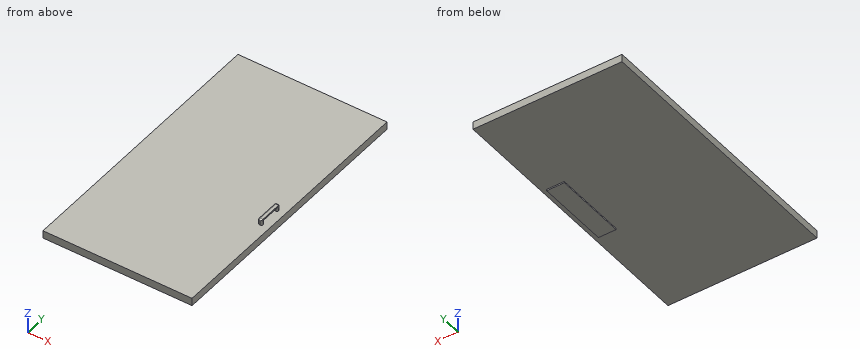
from build123d import *

# Parameters (mm, degrees)
BOSS_EXTRUDE2_DEPTH = 57.15
BOSS_EXTRUDE3_DEPTH = 44
CUT_EXTRUDE1_DEPTH  = 44
FILLET1_R           = 10
BOSS_EXTRUDE4_DEPTH = 10


with BuildPart() as part:
    # Sketch1 → Boss-Extrude2 (new body)
    with BuildSketch(Plane.XY):
        Polygon((0, 0), (0, 446.2018372120283), (-1100, 446.2018372120282), (-1100, -1585.7981627879717), (0, -1585.7981627879717), align=None)
    extrude(amount=BOSS_EXTRUDE2_DEPTH)

    # Sketch4 → Boss-Extrude3 (add)
    with BuildSketch(Plane.XY.offset(57.15)):
        Polygon((-79.99999999999993, -603.7981627879718), (-49.999999999999936, -603.7981627879718), (-49.999999999999915, -785.7981627879718), (-79.9999999999999, -785.7981627879718), align=None)
    extrude(amount=BOSS_EXTRUDE3_DEPTH)

    # Sketch5 → Cut-Extrude1 (cut)
    with BuildSketch(Plane.ZY.offset(80.00000000000003)):
        Polygon((83.14999999999999, -624.7981627879717), (57.150000000000006, -624.7981627879717), (57.15, -764.7981627879717), (83.15, -764.7981627879717), align=None)
    extrude(amount=-CUT_EXTRUDE1_DEPTH, mode=Mode.SUBTRACT)

    # Fillet1
    # the kernel refuses this fillet: 10 mm, written as the material it takes off along each edge
    with BuildSketch(Plane(origin=(-69.99999999999993, -613.7981627879718, 91.15), x_dir=(-1, -1.6e-16, 0), z_dir=(0, 1, 0))) as fillet1_piece_1_section:
        Polygon((0, 0), (FILLET1_R, 0), (FILLET1_R, FILLET1_R), (0, FILLET1_R), align=None)
    fillet1_piece_1 = extrude(amount=FILLET1_R, mode=Mode.PRIVATE)
    fillet1_piece_1 = fillet1_piece_1 - Plane(origin=(-69.99999999999993, -613.7981627879718, 91.15), x_dir=(0.7071067811865475, 0, -0.7071067811865475), z_dir=(0, 1, 0)) * Sphere(FILLET1_R, mode=Mode.PRIVATE)
    add(fillet1_piece_1, mode=Mode.SUBTRACT)
    with BuildSketch(Plane(origin=(-69.9999999999999, -775.7981627879718, 91.15), x_dir=(0, 0, 1), z_dir=(-1, -1.6e-16, 0))) as fillet1_piece_2_section:
        Polygon((0, 0), (FILLET1_R, 0), (FILLET1_R, -FILLET1_R), (0, -FILLET1_R), align=None)
    fillet1_piece_2 = extrude(amount=FILLET1_R, mode=Mode.PRIVATE)
    fillet1_piece_2 = fillet1_piece_2 - Plane(origin=(-69.9999999999999, -775.7981627879718, 91.15), x_dir=(0, 0.7071067811865475, -0.7071067811865475), z_dir=(-1, -1.6e-16, 0)) * Sphere(FILLET1_R, mode=Mode.PRIVATE)
    add(fillet1_piece_2, mode=Mode.SUBTRACT)
    with BuildSketch(Plane(origin=(-49.999999999999915, -785.7981627879718, 57.15), x_dir=(-1, 0, 0), z_dir=(0, 0, 1))) as fillet1_piece_3:
        with BuildLine():
            CenterArc((FILLET1_R, -FILLET1_R), FILLET1_R, 90, 90)
            Line((0, -FILLET1_R), (0, 0))
            Line((0, 0), (FILLET1_R, 0))
        make_face()
    extrude(amount=69, mode=Mode.SUBTRACT)
    with BuildSketch(Plane(origin=(-49.999999999999936, -603.7981627879718, 57.15), x_dir=(0, -1, 0), z_dir=(0, 0, 1))) as fillet1_piece_4:
        with BuildLine():
            CenterArc((FILLET1_R, -FILLET1_R), FILLET1_R, 90, 90)
            Line((0, -FILLET1_R), (0, 0))
            Line((0, 0), (FILLET1_R, 0))
        make_face()
    extrude(amount=69, mode=Mode.SUBTRACT)
    with BuildSketch(Plane(origin=(-79.99999999999993, -603.7981627879718, 57.15), x_dir=(1, 0, 0), z_dir=(0, 0, 1))) as fillet1_piece_5:
        with BuildLine():
            CenterArc((FILLET1_R, -FILLET1_R), FILLET1_R, 90, 90)
            Line((0, -FILLET1_R), (0, 0))
            Line((0, 0), (FILLET1_R, 0))
        make_face()
    extrude(amount=34.00000000000001, mode=Mode.SUBTRACT)
    with BuildSketch(Plane(origin=(-79.9999999999999, -785.7981627879718, 57.15), x_dir=(1, 0, 0), z_dir=(0, 0, 1))) as fillet1_piece_6:
        with BuildLine():
            CenterArc((FILLET1_R, FILLET1_R), FILLET1_R, 180, 90)
            Line((0, FILLET1_R), (0, 0))
            Line((0, 0), (FILLET1_R, 0))
        make_face()
    extrude(amount=34.00000000000001, mode=Mode.SUBTRACT)
    with BuildSketch(Plane(origin=(-69.99999999999993, -603.7981627879718, 101.15), x_dir=(0, 0, -1), z_dir=(1, 0, 0))) as fillet1_piece_7:
        with BuildLine():
            CenterArc((FILLET1_R, -FILLET1_R), FILLET1_R, 90, 90)
            Line((0, -FILLET1_R), (0, 0))
            Line((0, 0), (FILLET1_R, 0))
        make_face()
    extrude(amount=44.99999999999999, mode=Mode.SUBTRACT)
    with BuildSketch(Plane(origin=(-79.9999999999999, -775.7981627879718, 101.15), x_dir=(0, 0, -1), z_dir=(-1.6e-16, 1, 0))) as fillet1_piece_8:
        with BuildLine():
            CenterArc((FILLET1_R, -FILLET1_R), FILLET1_R, 90, 90)
            Line((0, -FILLET1_R), (0, 0))
            Line((0, 0), (FILLET1_R, 0))
        make_face()
    extrude(amount=162, mode=Mode.SUBTRACT)
    with BuildSketch(Plane(origin=(-24.999999999999915, -785.7981627879718, 101.15), x_dir=(0, 0, -1), z_dir=(-1, 0, 0))) as fillet1_piece_9:
        with BuildLine():
            CenterArc((FILLET1_R, -FILLET1_R), FILLET1_R, 90, 90)
            Line((0, -FILLET1_R), (0, 0))
            Line((0, 0), (FILLET1_R, 0))
        make_face()
    extrude(amount=44.999999999999986, mode=Mode.SUBTRACT)
    with BuildSketch(Plane(origin=(-79.99999999999991, -764.7981627879717, 57.15000000000002), x_dir=(1.42e-15, -1, 0), z_dir=(0, 0, 1))) as fillet1_piece_10:
        with BuildLine():
            CenterArc((FILLET1_R, FILLET1_R), FILLET1_R, 180, 89.99999999999989)
            Line((1.421e-14, FILLET1_R), (0, 0))
            Line((0, 0), (FILLET1_R, 0))
        make_face()
    extrude(amount=25.999999999999986, mode=Mode.SUBTRACT)
    with BuildSketch(Plane(origin=(-79.99999999999993, -624.7981627879717, 83.14999999999999), x_dir=(0, 1, 0), z_dir=(0, 0, -1))) as fillet1_piece_11:
        with BuildLine():
            CenterArc((FILLET1_R, FILLET1_R), FILLET1_R, 180, 90)
            Line((0, FILLET1_R), (0, 0))
            Line((0, 0), (FILLET1_R, 0))
        make_face()
    extrude(amount=25.999999999999986, mode=Mode.SUBTRACT)
    with BuildSketch(Plane(origin=(-79.99999999999991, -764.7981627879717, 83.15), x_dir=(1.42e-15, 1e-16, 1), z_dir=(-1.5e-16, 1, -1e-16))) as fillet1_piece_12:
        with BuildLine():
            CenterArc((FILLET1_R, FILLET1_R), FILLET1_R, 180, 89.99999999999989)
            Line((1.421e-14, FILLET1_R), (0, 0))
            Line((0, 0), (FILLET1_R, 0))
        make_face()
    extrude(amount=140, mode=Mode.SUBTRACT)
    with BuildSketch(Plane(origin=(-49.999999999999915, -764.7981627879717, 83.15), x_dir=(0, -1, 0), z_dir=(0, 0, -1))) as fillet1_piece_13:
        with BuildLine():
            CenterArc((FILLET1_R, FILLET1_R), FILLET1_R, 180, 90)
            Line((0, FILLET1_R), (0, 0))
            Line((0, 0), (FILLET1_R, 0))
        make_face()
    extrude(amount=26, mode=Mode.SUBTRACT)
    with BuildSketch(Plane(origin=(-49.999999999999936, -624.7981627879717, 57.150000000000006), x_dir=(0, 1, 0), z_dir=(0, 0, 1))) as fillet1_piece_14:
        with BuildLine():
            CenterArc((FILLET1_R, FILLET1_R), FILLET1_R, 180.00000000000003, 90)
            Line((0, FILLET1_R), (0, 0))
            Line((0, 0), (FILLET1_R, 0))
        make_face()
    extrude(amount=25.999999999999986, mode=Mode.SUBTRACT)
    with BuildSketch(Plane(origin=(-49.999999999999936, -624.7981627879717, 83.15), x_dir=(0, 1e-16, 1), z_dir=(1.2e-16, -1, 1e-16))) as fillet1_piece_15:
        with BuildLine():
            CenterArc((FILLET1_R, FILLET1_R), FILLET1_R, 180, 90)
            Line((0, FILLET1_R), (0, 0))
            Line((0, 0), (FILLET1_R, 0))
        make_face()
    extrude(amount=140, mode=Mode.SUBTRACT)
    with BuildSketch(Plane(origin=(-79.99999999999991, -764.7981627879717, 57.15000000000002), x_dir=(1.42e-15, -1, 0), z_dir=(0, 0, 1))) as fillet1_piece_16a_section:
        with BuildLine():
            CenterArc((FILLET1_R, FILLET1_R), FILLET1_R, 180, 89.99999999999989)
            Line((1.421e-14, FILLET1_R), (0, 0))
            Line((0, 0), (FILLET1_R, 0))
        make_face()
    fillet1_piece_16a = extrude(amount=50.999999999999986, mode=Mode.PRIVATE)
    fillet1_piece_16a = split(fillet1_piece_16a, bisect_by=Plane(origin=(-77.7360488573316, -767.0621139306398, 83.15), z_dir=(0, 1e-16, 1)), keep=Keep.TOP, mode=Mode.PRIVATE)
    with BuildSketch(Plane(origin=(-79.9999999999999, -789.7981627879717, 83.15), x_dir=(0, 1e-16, 1), z_dir=(-1.5e-16, 1, -1e-16))) as fillet1_piece_16b_section:
        with BuildLine():
            CenterArc((FILLET1_R, FILLET1_R), FILLET1_R, 180, 90)
            Line((0, FILLET1_R), (0, 0))
            Line((0, 0), (FILLET1_R, 0))
        make_face()
    fillet1_piece_16b = extrude(amount=165, mode=Mode.PRIVATE)
    fillet1_piece_16b = split(fillet1_piece_16b, bisect_by=Plane(origin=(-77.73604885733165, -764.7981627879717, 85.41395114266827), z_dir=(1.5e-16, -1, 0)), keep=Keep.TOP, mode=Mode.PRIVATE)
    fillet1_piece_16 = fillet1_piece_16a & fillet1_piece_16b
    add(fillet1_piece_16, mode=Mode.SUBTRACT)
    with BuildSketch(Plane(origin=(-79.99999999999991, -764.7981627879717, 83.15), x_dir=(1.42e-15, 1e-16, 1), z_dir=(-1.5e-16, 1, -1e-16))) as fillet1_piece_17a_section:
        with BuildLine():
            CenterArc((FILLET1_R, FILLET1_R), FILLET1_R, 180, 89.99999999999989)
            Line((1.421e-14, FILLET1_R), (0, 0))
            Line((0, 0), (FILLET1_R, 0))
        make_face()
    fillet1_piece_17a = extrude(amount=165, mode=Mode.PRIVATE)
    fillet1_piece_17a = split(fillet1_piece_17a, bisect_by=Plane(origin=(-77.73604885733167, -624.7981627879717, 85.41395114266825), z_dir=(-1.5e-16, 1, 0)), keep=Keep.TOP, mode=Mode.PRIVATE)
    with BuildSketch(Plane(origin=(-79.99999999999993, -624.7981627879717, 108.14999999999998), x_dir=(0, 1, 0), z_dir=(0, 0, -1))) as fillet1_piece_17b_section:
        with BuildLine():
            CenterArc((FILLET1_R, FILLET1_R), FILLET1_R, 180, 90)
            Line((0, FILLET1_R), (0, 0))
            Line((0, 0), (FILLET1_R, 0))
        make_face()
    fillet1_piece_17b = extrude(amount=50.999999999999986, mode=Mode.PRIVATE)
    fillet1_piece_17b = split(fillet1_piece_17b, bisect_by=Plane(origin=(-77.73604885733164, -622.5342116453035, 83.14999999999999), z_dir=(0, 1e-16, 1)), keep=Keep.TOP, mode=Mode.PRIVATE)
    fillet1_piece_17 = fillet1_piece_17a & fillet1_piece_17b
    add(fillet1_piece_17, mode=Mode.SUBTRACT)
    with BuildSketch(Plane(origin=(-49.999999999999936, -624.7981627879717, 83.15), x_dir=(0, 1e-16, 1), z_dir=(1.2e-16, -1, 1e-16))) as fillet1_piece_18a_section:
        with BuildLine():
            CenterArc((FILLET1_R, FILLET1_R), FILLET1_R, 180, 90)
            Line((0, FILLET1_R), (0, 0))
            Line((0, 0), (FILLET1_R, 0))
        make_face()
    fillet1_piece_18a = extrude(amount=165, mode=Mode.PRIVATE)
    fillet1_piece_18a = split(fillet1_piece_18a, bisect_by=Plane(origin=(-52.26395114266817, -764.7981627879717, 85.41395114266827), z_dir=(1.5e-16, -1, 0)), keep=Keep.TOP, mode=Mode.PRIVATE)
    with BuildSketch(Plane(origin=(-49.999999999999915, -764.7981627879717, 108.15), x_dir=(0, -1, 0), z_dir=(0, 0, -1))) as fillet1_piece_18b_section:
        with BuildLine():
            CenterArc((FILLET1_R, FILLET1_R), FILLET1_R, 180, 90)
            Line((0, FILLET1_R), (0, 0))
            Line((0, 0), (FILLET1_R, 0))
        make_face()
    fillet1_piece_18b = extrude(amount=51, mode=Mode.PRIVATE)
    fillet1_piece_18b = split(fillet1_piece_18b, bisect_by=Plane(origin=(-52.2639511426682, -767.0621139306397, 83.15), z_dir=(0, 1e-16, 1)), keep=Keep.TOP, mode=Mode.PRIVATE)
    fillet1_piece_18 = fillet1_piece_18a & fillet1_piece_18b
    add(fillet1_piece_18, mode=Mode.SUBTRACT)
    with BuildSketch(Plane(origin=(-49.999999999999936, -624.7981627879717, 57.150000000000006), x_dir=(0, 1, 0), z_dir=(0, 0, 1))) as fillet1_piece_19a_section:
        with BuildLine():
            CenterArc((FILLET1_R, FILLET1_R), FILLET1_R, 180.00000000000003, 90)
            Line((0, FILLET1_R), (0, 0))
            Line((0, 0), (FILLET1_R, 0))
        make_face()
    fillet1_piece_19a = extrude(amount=50.999999999999986, mode=Mode.PRIVATE)
    fillet1_piece_19a = split(fillet1_piece_19a, bisect_by=Plane(origin=(-52.26395114266823, -622.5342116453035, 83.14999999999999), z_dir=(0, 1e-16, 1)), keep=Keep.TOP, mode=Mode.PRIVATE)
    with BuildSketch(Plane(origin=(-49.999999999999936, -599.7981627879717, 83.14999999999999), x_dir=(0, 1e-16, 1), z_dir=(1.2e-16, -1, 1e-16))) as fillet1_piece_19b_section:
        with BuildLine():
            CenterArc((FILLET1_R, FILLET1_R), FILLET1_R, 179.99999999999997, 90)
            Line((0, FILLET1_R), (0, 0))
            Line((0, 0), (FILLET1_R, 0))
        make_face()
    fillet1_piece_19b = extrude(amount=165, mode=Mode.PRIVATE)
    fillet1_piece_19b = split(fillet1_piece_19b, bisect_by=Plane(origin=(-52.26395114266818, -624.7981627879717, 85.41395114266824), z_dir=(-1.5e-16, 1, 0)), keep=Keep.TOP, mode=Mode.PRIVATE)
    fillet1_piece_19 = fillet1_piece_19a & fillet1_piece_19b
    add(fillet1_piece_19, mode=Mode.SUBTRACT)

    # Sketch6 → Boss-Extrude4 (add)
    with BuildSketch(Plane(origin=(0, 0, 0), x_dir=(-1, 0, 0), z_dir=(0, 0, -1))):
        Polygon((34.99999999999994, -272.04870051020725), (164.99999999999986, -272.04870051020725), (165, -812.0487005102073), (35, -812.0487005102073), align=None)
    extrude(amount=BOSS_EXTRUDE4_DEPTH)


solid = part.part
CAD build for the part. Positions are in the model's coordinates, mm. Coordinates: 2 decimals unless noted, no trailing zeros. Write each loop counter-clockwise with the first axis right and the second up, starting at its lowest first coordinate (ties: lowest second). Pieces come first, ordered by that corner, then holes. Notation, with made-up numbers: (15.5, 46.25) - (60.5, 46.25) arc R34 cw to (60.5, 84.25) - close; hole circle Ø2 at (55, 31). An arc over 180 degrees is marked (long way). Use a Markdown table: item, result. Add a question column.
Item 1: Flat gauge pins, fed straight in: pin 1 (5 mm diameter, centred on y = -654, z = -3.5, fed in from +X); pin 2 (3 mm diameter, centred on x = -64.5, z = 65.5, fed in from -Y); pin 3 (8 mm diameter, centred on x = -66, z = 65, fed in from +Y); pin 4 (22 mm diameter, centred on y = -654.5, z = 68.5, fed in from +X). Where does each tip first touch, or does it go through?
Item 2: Band-saw the part on C-C, the plane y = -1294. Give the cut face in (x, z).
Item 3: Drill centre line: L1, parallel to Z at x = -301.5, y = -1237. Where is it in solid material? Low to high. Write a range as from..to.
Item 4: Band-saw the part on A-A, the plane y = -645.5. Give the cut face in (x, z), and give its area (3 significant figures).
Item 5: Band-saw the part on B-B, the plane x = -580. Give the cut face in (y, z).
Numbers:
| question | item | result |
|---|---|---|
| 1 | pin 1 | x = -35 |
| 1 | pin 2 | y = -785.8 |
| 1 | pin 3 | y = -603.8 |
| 1 | pin 4 | through |
| 2 | outline | (-1100, 0) - (0, 0) - (0, 57.15) - (-1100, 57.15) - close |
| 3 | L1 | 0..57.15 |
| 4 | outline | (-1100, 0) - (-165, 0) - (-165, -10) - (-35, -10) - (-35, 0) - (0, 0) - (0, 57.15) - (-1100, 57.15) - close; (-79.95, 92.15) arc R10 ccw to (-70, 83.15) - (-60, 83.15) arc R10 ccw to (-50, 93.15) - (-50, 101.15) - (-70, 101.15) arc R10 ccw to start |
| 4 | area | 64,600 mm2 |
| 5 | outline | (-1585.8, 0) - (446.2, 0) - (446.2, 57.15) - (-1585.8, 57.15) - close |
